Could you check a few things on this model? Use its own coordinates, in mm. Round coordinates to 2 decimals unless told otherwise and drop trailing zeros. Loops run counter-clockwise (first coordinate to the right, second up) from the corner with the lowest first, then second, coordinate; pieces in that order, holes last. Notation, with made-up numbers: (46, 77) -> (83, 77) arc R26 cw to (83, 110) -> close; hole circle Ø4 at (-23, -9). An arc over 180 degrees is marked (long way). Write each question's results on one line, items separated by ' | '.
Autodesk Inventor part; units mm, degrees
ref_plane "YZ Plane" through (0, 0, 0) normal (1, 0, 0) x (0, 1, 0)
ref_plane "XZ Plane" through (0, 0, 0) normal (0, 1, 0) x (-1, 0, 0)
ref_plane "XY Plane" through (0, 0, 0) normal (0, 0, 1) x (1, 0, 0)
sketch "Sketch8" plane through (0, 0, 0) normal (0, 0, 1) x (1, 0, 0)
  line L0 (0, 2897) -> (1200, 2897)
  line L1 (1200, 2897) -> (1200, 0)
  line L2 (1200, 0) -> (0, 0)
  line L3 (0, 0) -> (0, 2897)
  line L4 (0, 2897) -> (1200, 0) construction
  line L5 (1200, 2897) -> (0, 0) construction
  line L6 (947, 0) -> (1097, 150)
  line L7 (1097, 150) -> (1147, 2897)
  line L8 (0, 700) -> (1200, 700)
  line L9 (1112.5806, 1006) -> (837.057, 700)
  line L10 (110.253, 0) -> (110.253, 700)
  line L11 (796.688, 700) -> (1081.2157, 1016)
  line L12 (1081.2157, 1016) -> (1112.7627, 1016)
  point P0 (600, 1448.5)
  point P1 (1107.0109, 700)
  dimension "d43" = 1200
  dimension "d44" = 2897
  dimension "d45" = 53
  dimension "d46" = 947
  dimension "d47" = 150
  dimension "d48" = 103
  dimension "d49" = 700
  dimension "d55" = 306
  dimension "d57" = 110.253
  dimension "d61" = 48
  dimension "d65" = 10
  dimension "d66" = 30
extrude "Plate4" add sketch "Sketch8" against normal blind 3 contours L7 L9 L8 L11 L12 | L8 L7 L6 L2 L10 | L7 L8 L9
chamfer "Corner Chamfer1" distance 6 angle 45 2 edges at (947, 0, -1.5) (1097, 150, -1.5)
sketch "Sketch9" plane through (0, 0, 0) normal (0, 0, 1) x (1, 0, 0)
  line L0 (1097.1092, 155.999) -> (1092.7574, 145.7574)
  line L1 (1097.1092, 155.999) -> (1112.7627, 1016)
  line L2 (1112.7627, 1016) -> (1081.2157, 1016)
  line L3 (1081.2157, 1016) -> (796.688, 700)
  line L4 (796.688, 700) -> (110.253, 700)
  line L5 (110.253, 700) -> (110.253, 0)
  line L6 (110.253, 0) -> (941, 0)
  line L7 (951.2426, 4.2426) -> (941, 0)
  line L8 (951.2426, 4.2426) -> (1092.7574, 145.7574)
  circle A0 centre (130.253, 680) radius 5.5
  point P0 (0, 0)
  dimension "d67" = 11
  dimension "d68" = 20
  dimension "d69" = 20
extrude "Extrusion2" cut sketch "Sketch9" against normal through all contours A0
pattern_linear "Rectangular Pattern2" count 3 spacing 320 along (1, 0, 0) of "Extrusion2"
sketch "Sketch10" plane through (0, 0, 0) normal (0, 0, 1) x (1, 0, 0)
  circle A0 centre (770.253, 680) radius 5.5
  circle A1 centre (450.253, 680) radius 5.5
  circle A2 centre (130.253, 680) radius 5.5
  line L0 (1097.1092, 155.999) -> (1092.7574, 145.7574)
  line L1 (1097.1092, 155.999) -> (1112.7627, 1016)
  line L2 (1112.7627, 1016) -> (1081.2157, 1016)
  line L3 (1081.2157, 1016) -> (796.688, 700)
  line L4 (796.688, 700) -> (110.253, 700)
  line L5 (110.253, 700) -> (110.253, 0)
  line L6 (110.253, 0) -> (941, 0)
  line L7 (951.2426, 4.2426) -> (941, 0)
  line L8 (951.2426, 4.2426) -> (1092.7574, 145.7574)
  circle A3 centre (1072.2889, 983.6687) radius 5.5
  line L9 (1081.2157, 1016) -> (1112.254, 988.053)
  line L10 (1097.1092, 155.999) -> (1112.7627, 1016)
  point P0 (0, 0)
  dimension "d75" = 15
  dimension "d76" = 30
extrude "Extrusion3" cut sketch "Sketch10" against normal through all contours A3
equation "\"d50\" = Thickness"
equation "\"BendReliefWidth\" = Thickness"
equation "\"BendReliefDepth\" = 0.5 * Thickness"
equation "\"CornerReliefSize\" = 4 * Thickness"
equation "\"MinimumRemnant\" = 2 * Thickness"
equation "\"TransitionRadius\" = BendRadius"
equation "\"JacobiRadiusSize\" = BendRadius"
equation "\"GapSize\" = Thickness"
properties part number "BSH 015 board cone wall" material "09g2s"
1) I want a section at C-C, the plane y = 948.5. Write out the boundary of the cut face in (x, z), plus the area to 3 significant figures.
Model answer:
outline: (1020.44, -3) -> (1111.53, -3) -> (1111.53, 0) -> (1020.44, 0) -> close | area: 273 mm2
2) I'm going to push flat-ended pins straight in: pin 1 (1 mm diameter, centred on y = 739.5, z = -0.5, fed in from +X); pin 2 (1 mm diameter, centred on x = 519.5, z = -2, fed in from +Y); pin 3 (1.5 mm diameter, centred on y = 458.5, z = -1.5, fed in from +X). Where does each tip first touch, or does it pass through?
Model answer:
pin 1: stops at x = 1107.74 | pin 2: stops at y = 700 | pin 3: stops at x = 1102.63
3) I want a section at A-A, the plane z = -2.2. Write out the boundary of the cut face in (x, y), plus the area to 3 significant figures.
Model answer:
outline: (110.25, 0) -> (941, 0) -> (951.24, 4.24) -> (1092.76, 145.76) -> (1097.11, 156) -> (1112.76, 1016) -> (1081.22, 1016) -> (796.69, 700) -> (110.25, 700) -> close; hole circle Ø11 at (130.25, 680); hole circle Ø11 at (450.25, 680); hole circle Ø11 at (770.25, 680); hole circle Ø11 at (1072.29, 983.67) | area: 736,000 mm2
4) I need wall thicknesses on line 1 (X direction, y = 679, z = -2.6); line 2 (X direction, y = 680, z = -1.6); line 3 (Y direction, x = 735.5, z = -2.3). Which ranges of each line are inside material? Lowest first, please.
Model answer:
line 1: x = 110.25 to 124.84, 135.66 to 444.84, 455.66 to 764.84, 775.66 to 1106.63 | line 2: x = 110.25 to 124.75, 135.75 to 444.75, 455.75 to 764.75, 775.75 to 1106.65 | line 3: y = 0 to 700
5) I want a section at B-B, the plane x = 209.5. Write out the boundary of the cut face in (y, z).
Model answer:
outline: (0, -3) -> (700, -3) -> (700, 0) -> (0, 0) -> close
